```python
from build123d import *

# Parameters (mm, degrees)
PAD_DEPTH            = 16
POCKET_DEPTH         = 106.884114
POCKET_DEPTH_BACK    = 122.884114
POCKET001_DEPTH      = 0.001
POCKET001_DEPTH_BACK = 16.001


with BuildPart() as part:
    # Sketch → Pad (new body)
    with BuildSketch(Plane.XY):
        with BuildLine():
            ThreePointArc((4.949542, 31.272861), (3.097964, 33.964015), (0, 35))
            Line((0, -15), (0, 35))
            Line((0, -15), (5, -15))
            ThreePointArc((5, -15), (8.535534, -13.535534), (10, -10))
            Line((10, -10), (10, 13))
            ThreePointArc((10, 13), (9.951106, 13.69753), (9.805381, 14.381419))
            Line((4.949542, 31.272861), (9.805381, 14.381419))
        make_face()
    pad = extrude(amount=PAD_DEPTH)

    # Sketch001 → Pocket (cut, two sides)
    with BuildSketch(Plane.XY) as pocket_sk:
        with BuildLine():
            Line((0, 0), (5.05, 0))
            Line((5.05, 0), (5.05, 13.05))
            Line((5.05, 13.05), (0.144081, 29.991722))
            ThreePointArc((0.144081, 29.991722), (0.090116, 30.069913), (0, 30.1))
            Line((0, 30.1), (0, 0))
        make_face()
    pocket = extrude(amount=-POCKET_DEPTH, mode=Mode.SUBTRACT) + extrude(pocket_sk.sketch, amount=POCKET_DEPTH_BACK, mode=Mode.SUBTRACT)

    # Mirrored: Pad, Pocket across Sketch V_Axis
    add(pad.mirror(Plane(origin=(0, 0, 0), x_dir=(0, 0, 1), z_dir=(1, 0, 0))))
    add(pocket.mirror(Plane(origin=(0, 0, 0), x_dir=(0, 0, 1), z_dir=(1, 0, 0))), mode=Mode.SUBTRACT)

    # Sketch002 → Pocket001 (cut, two sides)
    with BuildSketch(Plane(origin=(-4, -6, 0), x_dir=(1, 0, 0), z_dir=(0, 0, 1))) as pocket001_sk:
        with BuildLine():
            ThreePointArc((3.55, 1.949359), (-4.05, 0), (3.55, -1.949359))
            Line((3.55, 1.949359), (3.55, -1.949359))
        make_face()
    extrude(amount=-POCKET001_DEPTH, mode=Mode.SUBTRACT)
    extrude(pocket001_sk.sketch, amount=POCKET001_DEPTH_BACK, mode=Mode.SUBTRACT)


solid = part.part
```
For this review, take the finished solid that the model builds, in its own axes (mm). A direction names the side the tool comes from. Round coordinates to 2 decimals unless told otherwise and drop trailing zeros. Write each loop counter-clockwise with the first axis right and the second up, starting at its lowest first coordinate (ties: lowest second). Pieces come first, ordered by that corner, then holes. Notation, with made-up numbers: M 35,-31.5 L 39,-31.5 A14 cw 39,-13.5 Z; hole C 36.25,59.5 d4. An arc over 180 degrees is marked long. One line per item, written item: value. Start each with the question number.
(1) Insertion check: pin 1 (2 mm diameter, centred on y = 23, z = 1.5, fed in from +X); pin 2 (8 mm diameter, centred on y = 20, z = 5, fed in from +X). Each pin has a flat end and moves straight along its axis. Give the tip position at first contact, or say it passes through.
(2) We need section A-A (y = -6). Give the boundary of the cut face in (x, z).
(3) Machinability: for faces 1 (the flat face through (10, 1, 8)), 2 (the flat face through (-0.45, -6, 8)), which of the approach directions +Z, -Z, +X, -X, +Y, -Y give a long, thin tool a straight path to every point of the face, cutting with its end or side? Answer none if there is none.
(4) The part is to be moulded in two halves that separate along Y. For faces 3 (the flat face through (7, 5, 0)), 4 (the cylindrical face through (-9.952, 13.688, 7.888)), 5 (the flat face through (-2.63, 21.4, 8.11)), say which applies: released by +Y, released by -Y, zero draft, split by the parting line, or undercut.
(5) Wall thickness on line 1 (X direction, y = -6, z = 11); line 2 (X direction, y = 5, z = 1.5); line 3 (X direction, y = -11, z = 13.75): over which ranges is each line inside the solid? List them lowest first.
(6) We need section D-D (y = 7). Give the boundary of the cut face in (x, z), and give its area (3 significant figures).
(7) We need section B-B (z = 14.25). Give the boundary of the cut face in (x, y).
(8) We need section C-C (x = -4). Give the boundary of the cut face in (y, z).
Result:
1. pin 1: x = 7.62
1. pin 2: x = 9.34
2. outline: M -10,0 L -8.05,0 L -8.05,16 L -10,16 Z; M -0.45,0 L 10,0 L 10,16 L -0.45,16 Z
3. face 1: +Z, -Z, +X, +Y, -Y
3. face 2: +Z, -Z
4. face 3: zero draft
4. face 4: released by +Y
4. face 5: undercut
5. line 1: -10 to -8.05, -0.45 to 10
5. line 2: -10 to -5.05, 5.05 to 10
5. line 3: -9.9 to 9.9
6. outline: M -10,0 L -5.05,0 L -5.05,16 L -10,16 Z; M 5.05,0 L 10,0 L 10,16 L 5.05,16 Z
6. area: 158 mm²
7. outline: M -10,-10 A5 ccw -5,-15 L 5,-15 A5 ccw 10,-10 L 10,13 A5 ccw 9.81,14.38 L 4.95,31.27 A5.15 ccw -4.95,31.27 L -9.81,14.38 A5 ccw -10,13 Z; hole M -5.05,0 L 5.05,0 L 5.05,13.05 L 0.14,29.99 A0.15 ccw -0.14,29.99 L -5.05,13.05 Z; hole M -0.45,-7.95 L -0.45,-4.05 A4.05 ccw long Z
8. outline: M -15,0 L -10.05,0 L -10.05,16 L -15,16 Z; M -1.95,0 L 0,0 L 0,16 L -1.95,16 Z; M 16.68,0 L 33.09,0 L 33.09,16 L 16.68,16 Z
